Geometry: see drawing. Coordinates: mm, zero at the bounding-box minimum. Coordinates: 2 decimals unless noted, no trailing zeros. Loops run counter-clockwise (first coordinate to the right, second up) from the corner with the lowest first, then second, coordinate; pieces in that order, holes last. Notation, with made-up numbers: (77, 51) - (81, 51) arc R9 cw to (81, 62) - close; hole circle Ø3 at (59, -31). An arc over 180 degrees is marked (long way). Answer in a Markdown table with one row per item.
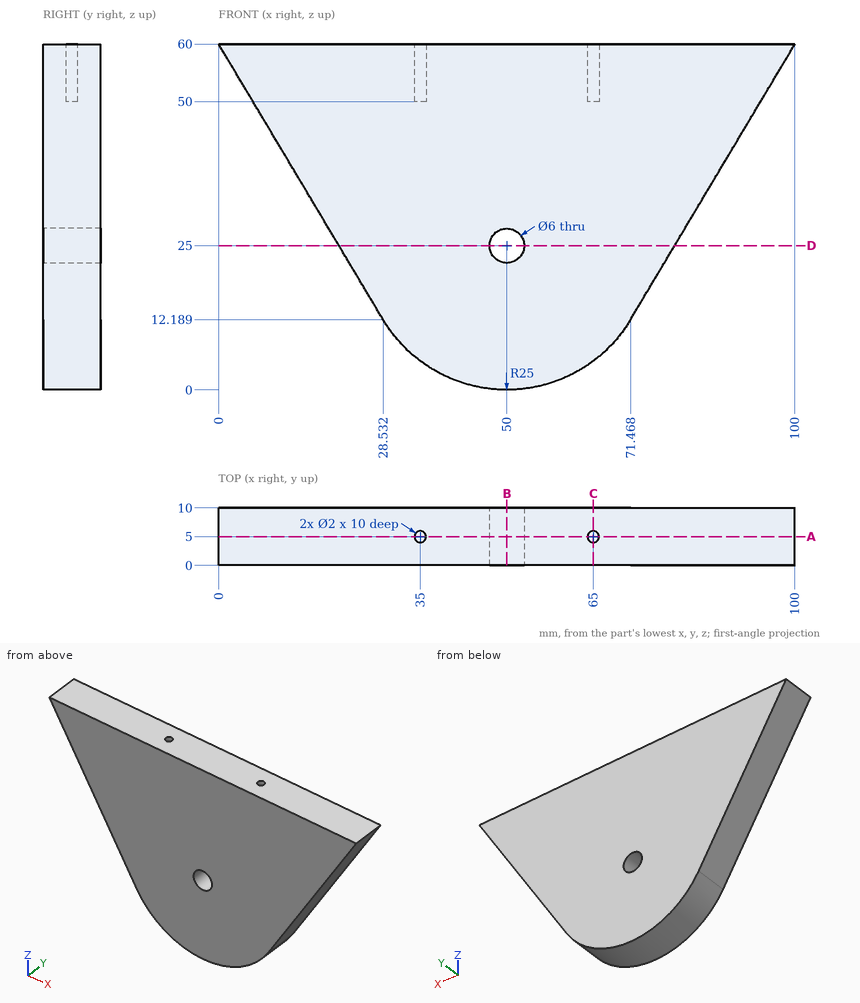
(1) Cut plane A-A on y = 5. Output: boundary loops of the cut face in (x, z), then the cut area to 3 significant figures.
Verdict:
| item | result |
|---|---|
| outline | (0, 60) - (28.53, 12.19) arc R25 ccw to (71.47, 12.19) - (100, 60) - (66, 60) - (66, 50) - (64, 50) - (64, 60) - (36, 60) - (36, 50) - (34, 50) - (34, 60) - close; hole circle Ø6 at (50, 25) |
| area | 3,720 mm² |
(2) Ray query, probe 1 along Y at (x, z) = (65, 55.5); probe 2 along Z at (x, y) = (51, 7); probe 3 along Z at (x, y) = (41, 8.75). Return the intervals inside material, ascending.
Verdict:
| item | result |
|---|---|
| probe 1 | y = 0 to 4, 6 to 10 |
| probe 2 | z = 0.02 to 22.17, 27.83 to 60 |
| probe 3 | z = 1.68 to 60 |
(3) Cut plane C-C on x = 65. Output: boundary loops of the cut face in (y, z), then the cut area to 3 significant figures.
Verdict:
| item | result |
|---|---|
| outline | (0, 5) - (10, 5) - (10, 60) - (6, 60) - (6, 50) - (4, 50) - (4, 60) - (0, 60) - close |
| area | 530 mm² |
(4) Cut plane D-D on z = 25. Output: boundary loops of the cut face in (x, y), then the cut area to 3 significant figures.
Verdict:
| item | result |
|---|---|
| outline | (20.89, 0) - (47, 0) - (47, 10) - (20.89, 10) - close; (53, 0) - (79.11, 0) - (79.11, 10) - (53, 10) - close |
| area | 522 mm² |
(5) First-contact query: pin 1 Ø6 at (y, z) = (1.5, 49) entering from -X; pin 2 Ø1 at (y, z) = (3.5, 14) entering from -X. Flat tips, straight axial feed; report the tip coordinate or a pass-through.
Verdict:
| item | result |
|---|---|
| pin 1 | stops at x = 4.77 |
| pin 2 | stops at x = 27.15 |
(6) Cut plane B-B on x = 50. Output: boundary loops of the cut face in (y, z), then the cut area to 3 significant figures.
Verdict:
| item | result |
|---|---|
| outline | (0, 0) - (10, 0) - (10, 22) - (0, 22) - close; (0, 28) - (10, 28) - (10, 60) - (0, 60) - close |
| area | 540 mm² |
